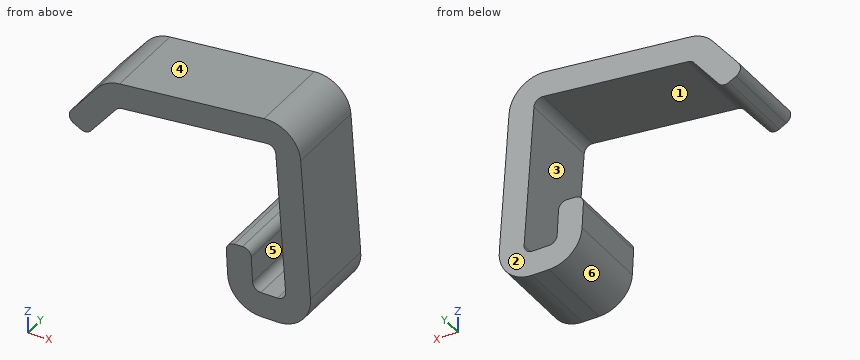
```python
from build123d import *

# Parameters (mm, degrees)
F1_DEPTH = 10
F2_R     = 1
F3_R     = 4


# Not quite as in the source:
# - two fillets or chamfers of one size are made in one step
# - a feature names something its author has since deleted; it is built from what else it names


with BuildPart() as f1:
    # F0 (on Front) → F1 (new body)
    with BuildSketch(Plane.XZ):
        Polygon((30.9209997221, 8.3203603271), (30.6589608257, 13.3203603271), (27.6630722214, 13.1633524584), (28.0741060219, 5.3203603271), (38.1381058522, 5.3203603271), (36.3716140423, 30.5823701452), (13.2265466485, 28.1497255366), (8.2771753479, 22.0377609909), (10.9237883626, 20.6251607112), (14.6997107089, 25.28803648), (33.5956267209, 27.274077282), (34.9209997221, 8.3203603271), align=None)
    extrude(amount=F1_DEPTH)

    # F2
    f2_edges = [f1.edges().sort_by_distance(p)[0] for p in [
        (34.921, -5, 8.32036),
        (30.921, -5, 8.32036),
        (14.699711, -5, 25.288036),
        (8.277175, -5, 22.037761),
        (10.923788, -5, 20.625161),
        (33.595627, -5, 27.274077),
        (30.658961, -5, 13.32036),
        (27.663072, -5, 13.163352),
    ]]
    fillet(f2_edges, radius=F2_R)

    # F3
    f3_edges = [f1.edges().sort_by_distance(p)[0] for p in [
        (38.138106, -5, 5.32036),
        (28.074106, -5, 5.32036),
        (13.226547, -5, 28.149726),
        (36.371614, -5, 30.58237),
    ]]
    fillet(f3_edges, radius=F3_R)


solid = f1.part
```
Could you check a few things on this model? Use its own coordinates, in mm. Face numbers are marked on the shaded views. A direction names the side the tool comes from. Give positions to 0.01 mm unless a question says otherwise; leave off trailing zeros. Order: outer loops, then holes, each group sorted by start corner. A loop starts at its lowest first (then second) coordinate and runs counter-clockwise, first axis right, second up.
Q1. Suppose I cut it at C-C, the plane y = -2.75. Write out the boundary of the cut face in (x, z).
Q2. Suppose I cut it at A-A, the plane z = 24.25. Write out the boundary of the cut face in (x, y), and give its area (3 significant figures).
Q3. I'm going to push flat-ended pins straight in: P1, Ø3, axis at y = -8.5, z = 25.5, coming from the +X side; P2, Ø0.6, axis at x = 33.5, y = -4, coming from the +Z side; P3, Ø3, axis at x = 24, y = -2, coming from the +Z side; P4, Ø12, axis at x = 24.5, z = 13.5, coming from the -Y side. Where does each tip first touch, or does it pass through?
Q4. For the marked faces 5 and 6, which set-ups out of +Z, -Z, +X, -X, +Y, -Y let a thin tool reach every point of the face, with its end or its side?
Q5. Suppose I cut it at B-B, the plane x = 33. Write out the boundary of the cut face in (y, z), and give its area (3 significant figures).
Q6. If I drill on line 1 along Z through (x, y) = (32.75, -3.75); line 2 along X through (y, z) = (-8, 13); line 3 along Z through (x, y) = (30.5, -4.75), over which ranges is the centre line in solid material (lowest first)?
Q7. We'd pull the mould along Z, two halves only. Please class the marked faces 1, 2, 3 and 4: +Z half, -Z half, draft (parallel to the pull), parting line (faces both ways), or undercut.
Q8. Suppose I cut it at D-D, the plane x = 19.5. Write out the boundary of the cut face in (y, z).
Solution:
1. outline: (9.04, 22.98) arc R1 ccw to (9.35, 21.47) - (10.2, 21.01) arc R1 ccw to (11.44, 21.27) - (14.44, 24.97) arc R1 cw to (15.11, 25.33) - (32.57, 27.17) arc R1 cw to (33.67, 26.24) - (34.85, 9.39) arc R1 cw to (33.85, 8.32) - (31.87, 8.32) arc R1 cw to (30.87, 9.27) - (30.71, 12.32) arc R1 ccw to (29.66, 13.27) - (28.66, 13.22) arc R1 ccw to (27.72, 12.16) - (27.88, 9.11) arc R4 ccw to (31.87, 5.32) - (33.85, 5.32) arc R4 ccw to (37.84, 9.6) - (36.66, 26.45) arc R4 ccw to (32.25, 30.15) - (14.87, 28.32) arc R4 ccw to (12.18, 26.86) - close
2. outline: (10.07, -10) - (13.86, -10) - (13.86, 0) - (10.07, 0) - close; (33.81, -10) - (36.81, -10) - (36.81, 0) - (33.81, 0) - close
2. area: 68.0 mm2
3. P1: stops at x = 36.83
3. P2: stops at z = 30.14
3. P3: stops at z = 29.44
3. P4: stops at y = -10
4. face 5: +Y, -Y
4. face 6: -Z, -X, +Y, -Y
5. outline: (-10, 5.32) - (0, 5.32) - (0, 8.32) - (-10, 8.32) - close; (-10, 27.12) - (0, 27.12) - (0, 30.16) - (-10, 30.16) - close
5. area: 60.4 mm2
6. line 1: z = 5.32 to 8.32, 27.17 to 30.17
6. line 2: x = 28.09 to 30.4, 34.59 to 37.6
6. line 3: z = 5.56 to 12.89, 26.95 to 29.97
7. face 1: undercut
7. face 2: draft
7. face 3: undercut
7. face 4: +Z half
8. outline: (-10, 25.79) - (0, 25.79) - (0, 28.81) - (-10, 28.81) - close
